Geometry check sheet. Reference: the model listing, model coordinates, mm. A direction names the side the tool comes from. Give positions to 0.01 mm unless a question says otherwise; leave off trailing zeros. Write each loop counter-clockwise with the first axis right and the second up, starting at its lowest first coordinate (ties: lowest second). Pieces come first, ordered by that corner, then holes. Notation, with made-up numbers: (2.5, 69) - (42.5, 69) arc R16 cw to (42.5, 74) - close; hole circle Ø7 at (2, 83). An arc over 180 degrees is marked (long way). One line per question, with ' | ' between items. Start each with the question number.
Q1. Section check A-A on y = 46.5. Record the boundary of the cut face in (x, z).
Q2. Section check D-D on y = 102.5. Record the boundary of the cut face in (x, z), and give its area (3 significant figures).
Q3. Section check B-B on x = 27.5. Record the boundary of the cut face in (y, z).
Q4. Gauge pin test, flat ends, axial feed: P1, Ø8, axis at x = 24.5, z = 5.5, coming from the +Y side; P2, Ø10, axis at x = 34, y = 63.5, coming from the +Z side; P3, Ø5, axis at x = 70.5, z = 24.5, coming from the +Y side; P4, Ø5, axis at y = 8.5, z = 3, coming from the -X side. Record the tip position at first contact, or that the pin passes through.
Q5. Set-up check for faces 4 (the face through (3, 90.8, 5)), 5 (the face through (37, 65.8, 5)), 6 (the face through (72, 40.4, 20)), 7 (the face through (6.5, 12, 5)), 8 (the face through (68.5, 45, 11)): record each of +Z, -Z, +X, -X, +Y, -Y from which the full face is reachable in a straight line by a thin tool's end or side.
Q6. Release check for a two-part mould opening along X. For faces 1 (the face through (75, 62, 7)), 2 (the face through (3, 0, 5)), 3 (the face through (6.5, 45, 11)) record: +X half, -X half, draft (parallel to the pull), parting line (faces both ways), or undercut.
Q7. Thickness scan on L1, parallel to X at y = 45.5, z = 27; L2, parallel to Y at x = 64.5, z = 3.5; L3, parallel to X at y = 105, z = 7.25. Record the ranges inside material, lowest first. Write a range as [from, to].
Q8. Section check C-C on z = 7.5. Record the boundary of the cut face in (x, y), and give its area (3 significant figures).
```python
from build123d import *

# Parameters (mm, degrees)
SKETCH1_W           = 6.5
SKETCH1_H           = 90.8
SKETCH1_H_2         = 135.4
SKETCH1_W_2         = 62
SKETCH1_H_3         = 6.5
BOSS_EXTRUDE1_DEPTH = 10
SKETCH2_W           = 6.5
SKETCH2_H           = 10
BOSS_EXTRUDE2_DEPTH = 20


with BuildPart() as part:
    # Sketch1 → Boss-Extrude1 (new body)
    with BuildSketch(Plane.XY):
        with Locations((3.25, 45.4)):
            Rectangle(SKETCH1_W, SKETCH1_H)
        with Locations((71.75, 67.7)):
            Rectangle(SKETCH1_W, SKETCH1_H_2)
        with Locations((37.5, 28.25)):
            Rectangle(SKETCH1_W_2, SKETCH1_H_3)
        with Locations((37.5, 62.55)):
            Rectangle(SKETCH1_W_2, SKETCH1_H_3)
    extrude(amount=BOSS_EXTRUDE1_DEPTH)

    # Sketch2 → Boss-Extrude2 (add)
    with BuildSketch(Plane.XY.offset(10)):
        with Locations((3.25, 45.4)):
            Rectangle(SKETCH2_W, SKETCH2_H)
        with Locations((71.75, 45.4)):
            Rectangle(SKETCH2_W, SKETCH2_H)
    extrude(amount=BOSS_EXTRUDE2_DEPTH)


solid = part.part
```
Working result:
1) outline: (0, 0) - (6.5, 0) - (6.5, 30) - (0, 30) - close; (68.5, 0) - (75, 0) - (75, 30) - (68.5, 30) - close
2) outline: (68.5, 0) - (75, 0) - (75, 10) - (68.5, 10) - close | area: 65.0 mm2
3) outline: (25, 0) - (31.5, 0) - (31.5, 10) - (25, 10) - close; (59.3, 0) - (65.8, 0) - (65.8, 10) - (59.3, 10) - close
4) P1: stops at y = 65.8 | P2: stops at z = 10 | P3: stops at y = 50.4 | P4: stops at x = 0
5) face 4: +Z, -Z, -X, +Y | face 5: +Z, -Z, +Y | face 6: +Z, +X, -X, -Y | face 7: +Z, -Z, -Y | face 8: +Z, -Z
6) face 1: +X half | face 2: draft | face 3: undercut
7) L1: x = [0, 6.5], [68.5, 75] | L2: y = [25, 31.5], [59.3, 65.8] | L3: x = [68.5, 75]
8) outline: (0, 0) - (6.5, 0) - (6.5, 25) - (68.5, 25) - (68.5, 0) - (75, 0) - (75, 135.4) - (68.5, 135.4) - (68.5, 65.8) - (6.5, 65.8) - (6.5, 90.8) - (0, 90.8) - close; hole (6.5, 31.5) - (68.5, 31.5) - (68.5, 59.3) - (6.5, 59.3) - close | area: 2,280 mm2
